```python
from build123d import *

# Parameters (mm, degrees)
F0_R     = 50.8
F1_DEPTH = 12.7
F3_DEPTH = 1752.6


with BuildPart() as f1:
    # F0 (on Top) → F1 (new body)
    with BuildSketch(Plane.XY):
        Circle(F0_R)
    extrude(amount=F1_DEPTH)

    # F2 (on face) → F3 (join)
    with BuildSketch(Plane.XY.offset(12.7)):
        with BuildLine():
            ThreePointArc((-0.0031752568, -20.9190722188), (-0.0312761161, -21.0825451789), (-0.06148119, -21.245642452))
            ThreePointArc((-0.06148119, -21.245642452), (-0.0031888656, -21.2456971257), (0.055103468, -21.2456532358))
            ThreePointArc((0.055103468, -21.2456532358), (0.024912457, -21.0825503951), (-0.0031752568, -20.9190722188))
        make_face()
        with BuildLine():
            ThreePointArc((23.5776117563, -11.9227459757), (31.6337017768, -0.4762724508), (34.4751987068, 13.2295014337))
            ThreePointArc((34.4751987068, 13.2295014337), (-13.7086998604, 44.861935327), (-23.5729583189, -11.92710728))
            ThreePointArc((-23.5729583189, -11.92710728), (-10.1369376903, -6.2068210975), (-0.0031752568, -16.7213435918))
            ThreePointArc((-0.0031752568, -16.7213435918), (10.1345978143, -6.2009032292), (23.5776117563, -11.9227459757))
        make_face()
        with BuildLine():
            ThreePointArc((-0.0031752568, -16.7213435918), (-10.1369376903, -6.2068210975), (-23.5729583189, -11.92710728))
            ThreePointArc((-23.5729583189, -11.92710728), (-12.7025767923, -18.8202079053), (-0.06148119, -21.245642452))
            ThreePointArc((-0.06148119, -21.245642452), (-0.0312761161, -21.0825451789), (-0.0031752568, -20.9190722188))
            ThreePointArc((-0.0031752568, -20.9190722188), (-0.1753642908, -18.8202079053), (-0.0031752568, -16.7213435918))
        make_face()
        with BuildLine():
            ThreePointArc((0.055103468, -21.2456532358), (12.7025767923, -18.8202079053), (23.5776117563, -11.9227459757))
            ThreePointArc((23.5776117563, -11.9227459757), (10.1345978143, -6.2009032292), (-0.0031752568, -16.7213435918))
            ThreePointArc((-0.0031752568, -16.7213435918), (0.1259579382, -17.7672466366), (0.1690987306, -18.8202079053))
            ThreePointArc((0.1690987306, -18.8202079053), (0.1259579382, -19.873169174), (-0.0031752568, -20.9190722188))
            ThreePointArc((-0.0031752568, -20.9190722188), (0.024912457, -21.0825503951), (0.055103468, -21.2456532358))
        make_face()
    extrude(amount=F3_DEPTH)


solid = f1.part
```
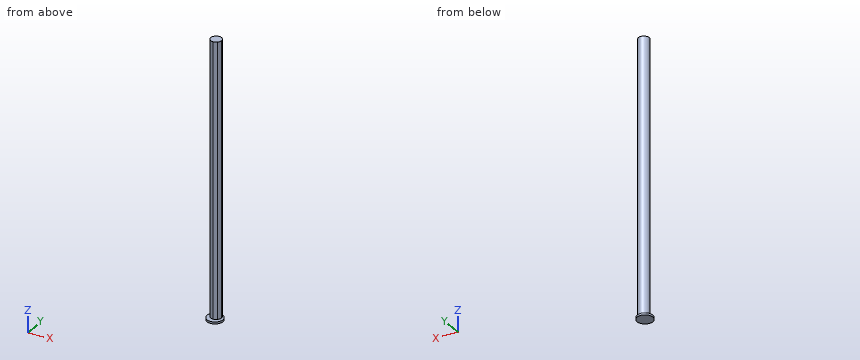
For this review, take the finished solid that the model builds, in its own axes (mm). Round coordinates to 2 decimals unless told otherwise and drop trailing zeros. Write each loop counter-clockwise with the first axis right and the second up, starting at its lowest first coordinate (ties: lowest second). Pieces come first, ordered by that corner, then holes. Notation, with made-up numbers: (72, -35) - (120, -35) arc R30 ccw to (120, -8) - close; hole circle Ø2 at (-2.75, 65.25). An arc over 180 degrees is marked (long way). Answer as a JSON object with one key per item and string values.
1. To check wall thickness, follow line 1 along X through (y, z) = (9.5, 1661); line 2 along Z through (x, y) = (44, -9); line 3 along Y through (x, z) = (-0.5, 666.5). State the ranges of each line that lie inside material, in increasing order.
Response values:
{"line 1": "x = -34.27 to 34.27", "line 2": "z = 0 to 12.7", "line 3": "y = -21.24 to 47.7"}
2. For pin 1 Ø2 at (y, z) = (22.5, 654.5) entering from +X; pin 2 Ø5 at (y, z) = (22, 270) entering from +X; pin 3 Ø10 at (x, z) = (36, 1017) entering from -Y, all flat-tipped, find the tip position at first contact; note any pin that passes through.
Response values:
{"pin 1": "stops at x = 33.47", "pin 2": "stops at x = 33.9", "pin 3": "stops at y = -1.85"}
3. We need section A-A on z = 1441.5. Give the boundary of the cut face in (x, y), then the cut area to 3 significant figures.
Response values:
{"outline": "(-0.06, -21.25) arc R34.48 ccw to (0.06, -21.25) arc R34.48 ccw (long way) to start; hole (0, -20.92) arc R12.87 ccw to (0, -16.72) arc R12.88 ccw to start", "area": "3,730 mm2"}
